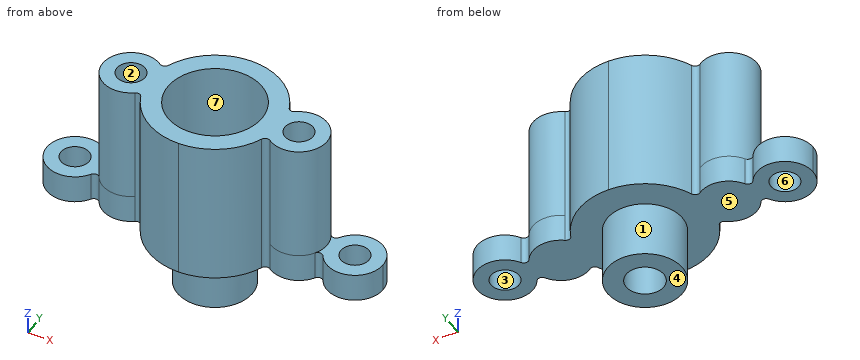
```python
from build123d import *

# Parameters (mm, degrees)
F1_DEPTH = 3
F2_R     = 1.5
F3_DEPTH = 12.5
F4_R     = 4
F4_R_2   = 2
F5_DEPTH = 6


with BuildPart() as f1:
    # F0 (on Top) → F1 (new body)
    with BuildSketch(Plane.XY):
        with BuildLine():
            ThreePointArc((7.238095, 2.428105), (6.807286, 2.351969), (6.481481, 2.643936))
            ThreePointArc((6.481481, 2.643936), (3.904641, 5.8098), (0, 7))
            ThreePointArc((0, 7), (-3.904641, 5.8098), (-6.481481, 2.643936))
            ThreePointArc((-6.481481, 2.643936), (-6.807286, 2.351969), (-7.238095, 2.428105))
            ThreePointArc((-7.238095, 2.428105), (-9.598913, 2.939609), (-11.571429, 1.545236))
            ThreePointArc((-11.571429, 1.545236), (-12, 1.302776), (-12.428571, 1.545236))
            ThreePointArc((-12.428571, 1.545236), (-15.801784, 2.890872), (-18, 0))
            ThreePointArc((-18, 0), (-15.801784, -2.890872), (-12.428571, -1.545236))
            ThreePointArc((-12.428571, -1.545236), (-12, -1.302776), (-11.571429, -1.545236))
            ThreePointArc((-11.571429, -1.545236), (-9.598913, -2.939609), (-7.238095, -2.428105))
            ThreePointArc((-7.238095, -2.428105), (-6.807286, -2.351969), (-6.481481, -2.643936))
            ThreePointArc((-6.481481, -2.643936), (-3.904641, -5.8098), (0, -7))
            ThreePointArc((0, -7), (3.904641, -5.8098), (6.481481, -2.643936))
            ThreePointArc((6.481481, -2.643936), (6.807286, -2.351969), (7.238095, -2.428105))
            ThreePointArc((7.238095, -2.428105), (9.598913, -2.939609), (11.571429, -1.545236))
            ThreePointArc((11.571429, -1.545236), (12, -1.302776), (12.428571, -1.545236))
            ThreePointArc((12.428571, -1.545236), (15.801784, -2.890872), (18, 0))
            ThreePointArc((18, 0), (15.801784, 2.890872), (12.428571, 1.545236))
            ThreePointArc((12.428571, 1.545236), (12, 1.302776), (11.571429, 1.545236))
            ThreePointArc((11.571429, 1.545236), (9.598913, 2.939609), (7.238095, 2.428105))
        make_face()
        with BuildLine():
            ThreePointArc((-16.5, 0), (-15, 1.5), (-13.5, 0))
            ThreePointArc((-13.5, 0), (-15, -1.5), (-16.5, 0))
        make_face(mode=Mode.SUBTRACT)
        with BuildLine():
            ThreePointArc((0, -1.5), (-1.5, 0), (0, 1.5))
            ThreePointArc((0, 1.5), (1.5, 0), (0, -1.5))
        make_face(mode=Mode.SUBTRACT)
        with BuildLine():
            ThreePointArc((16.5, 0), (15, -1.5), (13.5, 0))
            ThreePointArc((13.5, 0), (15, 1.5), (16.5, 0))
        make_face(mode=Mode.SUBTRACT)
    extrude(amount=F1_DEPTH)

    # F2 (on face) → F3 (join)
    with BuildSketch(Plane.XY.offset(3)):
        with BuildLine():
            ThreePointArc((7.238095, 2.428105), (6.807286, 2.351969), (6.481481, 2.643936))
            ThreePointArc((6.481481, 2.643936), (3.904641, 5.8098), (0, 7))
            ThreePointArc((0, 7), (-3.904641, 5.8098), (-6.481481, 2.643936))
            ThreePointArc((-6.481481, 2.643936), (-6.807286, 2.351969), (-7.238095, 2.428105))
            ThreePointArc((-7.238095, 2.428105), (-12, 0), (-7.238095, -2.428105))
            ThreePointArc((-7.238095, -2.428105), (-6.807286, -2.351969), (-6.481481, -2.643936))
            ThreePointArc((-6.481481, -2.643936), (-3.904641, -5.8098), (0, -7))
            ThreePointArc((0, -7), (3.904641, -5.8098), (6.481481, -2.643936))
            ThreePointArc((6.481481, -2.643936), (6.807286, -2.351969), (7.238095, -2.428105))
            ThreePointArc((7.238095, -2.428105), (12, 0), (7.238095, 2.428105))
        make_face()
        with Locations((-9, 0)):
            Circle(F2_R, mode=Mode.SUBTRACT)
        with BuildLine():
            ThreePointArc((0, -5), (-5, 0), (0, 5))
            ThreePointArc((0, 5), (5, 0), (0, -5))
        make_face(mode=Mode.SUBTRACT)
        with Locations((9, 0)):
            Circle(F2_R, mode=Mode.SUBTRACT)
    extrude(amount=F3_DEPTH)

    # F4 (on face) → F5 (join)
    with BuildSketch(Plane.XY):
        Circle(F4_R)
        Circle(F4_R_2, mode=Mode.SUBTRACT)
    extrude(amount=-F5_DEPTH)


solid = f1.part
```
Geometry: final body of the model. Coordinates: model frame, mm. Face numbers are marked on the shaded views. A direction names the side the tool comes from. Round coordinates to 2 decimals unless told otherwise and drop trailing zeros. Write each loop counter-clockwise with the first axis right and the second up, starting at its lowest first coordinate (ties: lowest second). Pieces come first, ordered by that corner, then holes.
Item 1: Material intervals for L1, parallel to Y at x = 15, z = 0.75; L2, parallel to X at y = 0.5, z = 9.25; L3, parallel to Y at x = 0, z = -3.3, sorted ascending.
Item 2: Section query A-A (x = 15). Return loops of the section in (y, z), plus the area to 3 significant figures.
Item 3: Mould query, pull axis X, two halves, no side actions, for the marked faces 1, 2, 3 and 4. Classes: +X half, -X half, draft (parallel to the pull), parting line (faces both ways), or undercut.
Item 4: Set-up query: the marked faces 5, 6 and 7. Return all of +Z, -Z, +X, -X, +Y, -Y with unobstructed straight access to the full face (end or side cutting, diameter ignored); none if empty.
Item 5: Section query D-D (z = -0.75). Return loops of the section in (x, y).
Item 6: Section query C-C (x = 9). Return loops of the section in (y, z), plus the area to 3 significant figures.
Item 7: Pin query (flat end, axial travel): P1, Ø6, axis at y = 2.5, z = 12, coming from the -X side; P2, Ø4, axis at x = -15, y = 0, coming from the +Z side; P3, Ø4, axis at y = 2, z = 7, coming from the +X side. Return the tip coordinate at first contact, or that it passes through.
Item 8: Section query B-B (z = 8.5). Return loops of the section in (x, y), plus the area to 3 significant figures.
Completed:
1. L1: y = -3 to -1.5, 1.5 to 3
1. L2: x = -11.96 to -10.41, -7.59 to -4.97, 4.97 to 7.59, 10.41 to 11.96
1. L3: y = -4 to -2, 2 to 4
2. outline: (-3, 0) - (-1.5, 0) - (-1.5, 3) - (-3, 3) - close; (1.5, 0) - (3, 0) - (3, 3) - (1.5, 3) - close
2. area: 9.00 mm2
3. face 1: parting line
3. face 2: undercut
3. face 3: undercut
3. face 4: draft
4. face 5: -Z
4. face 6: +Z, -Z
4. face 7: +Z
5. outline: circle Ø8 at (0, 0); hole circle Ø4 at (0, 0)
6. outline: (-3, 0) - (3, 0) - (3, 15.5) - (1.5, 15.5) - (1.5, 3) - (-1.5, 3) - (-1.5, 15.5) - (-3, 15.5) - close
6. area: 55.5 mm2
7. P1: stops at x = -12
7. P2: stops at z = 3
7. P3: stops at x = 12
8. outline: (-7.24, -2.43) arc R0.5 cw to (-6.48, -2.64) arc R7 ccw to (6.48, -2.64) arc R0.5 cw to (7.24, -2.43) arc R3 ccw (long way) to (7.24, 2.43) arc R0.5 cw to (6.48, 2.64) arc R7 ccw to (-6.48, 2.64) arc R0.5 cw to (-7.24, 2.43) arc R3 ccw (long way) to start; hole circle Ø3 at (-9, 0); hole circle Ø10 at (0, 0); hole circle Ø3 at (9, 0)
8. area: 113 mm2
